from build123d import *

# Parameters (mm, degrees)
CHAMFER_1_SIZE = 1
CHAMFER_2_SIZE = 1
FILLET_1_R     = 0.2


with BuildPart() as part:
    # 스케치3 → 회전2 (revolve)
    with BuildSketch(Plane(origin=(0, 0, 0), x_dir=(1, 0, 0), z_dir=(0, 1, 0)), mode=Mode.PRIVATE) as revolve_2_sk:
        Polygon((11.1, 0), (11.1, -2.4), (8.6, -2.4), (8.6, -4.2), (11.1, -6.2), (11.1, -8.2), (10, -8.2), (10, -10.2), (9.5, -10.7), (9.5, -11.2), (10, -11.7), (10, -12.2), (9.5, -12.7), (9.5, -13.2), (10, -13.7), (10, -14.2), (9.5, -14.7), (9.5, -15.2), (10, -15.7), (10, -16.2), (9.5, -16.7), (9.5, -17.2), (10, -17.7), (10, -19.8), (2.9, -19.8), (2.9, -11.8), (4.4, -11.8), (4.4, -10), (3.4, -10), (3.4, -8.5), (6.25, -7.736344802), (6.25, 0), align=None)
    revolve(revolve_2_sk.sketch.rotate(Axis((0, 0, 0), (0, 0, 1)), 180), axis=Axis((0, 0, 0), (0, 0, 1)))

    # 모따기1
    chamfer_1_edges = [part.edges().sort_by_distance(p)[0] for p in [
        (10, 0, 19.8),
        (6.25, 0, 0),
    ]]
    chamfer(chamfer_1_edges, length=CHAMFER_1_SIZE)

    # 모따기2
    chamfer_2_edges = [part.edges().sort_by_distance(p)[0] for p in [
        (11.1, 0, 0),
    ]]
    chamfer(chamfer_2_edges, length=CHAMFER_2_SIZE)

    # 필렛1
    fillet_1_edges = [part.edges().sort_by_distance(p)[0] for p in [
        (11.1, 0, 2.4),
    ]]
    fillet(fillet_1_edges, radius=FILLET_1_R)


solid = part.part
Could you check a few things on this model? Use its own coordinates, in mm. A direction names the side the tool comes from. Give positions to 0.01 mm unless a question says otherwise; leave off trailing zeros. Write each loop counter-clockwise with the first axis right and the second up, starting at its lowest first coordinate (ties: lowest second). Pieces come first, ordered by that corner, then holes. Notation, with made-up numbers: (-25, 23.25) -> (-6, 23.25) arc R26 cw to (-6, 45.25) -> close; hole circle Ø1 at (-33.75, -15.5). An arc over 180 degrees is marked (long way). Answer as CSV lines item,"result". Start each with the question number.
(1) I'm going to push flat-ended pins straight in: pin 1 Ø5 at (y, z) = (8, 11.5) entering from -X; pin 2 Ø5 at (y, z) = (-7, 14.5) entering from -X; pin 3 Ø4.5 at (x, y) = (2, 1.5) entering from -Z. Where does each tip first touch, or does it pass through?
(2) Which directions (+Z, -Z, +X, -X, +Y, -Y) give clear straight access to the entire face, cutting with the end or side of a thin tool? Please do faces 4 (the face through (1.445, -11.006, 7.214)), 5 (the face through (10, 0, 14)), 6 (the face through (-5.96, -1.88, 4.32)), 7 (the face through (2.059, 9.274, 16.954)).
(3) If we section it at A-A, the plane z = 5: Write out the boundary of the cut face in (x, y), and give its area (3 significant figures).
(4) If we mould it in two halves opening along X, with no side actions, what happens to faces 1 (the face through (0.74, 3.32, 9.24)), 2 (the face through (10, 0, 18)), 3 (the face through (0, 4, 19.8))? For each: +X half, -X half, draft (parallel to the pull), parting line (faces both ways), or undercut.
(5) Please list where these lines run through material, in increasing order: line 1 (Y direction, x = 0, z = 9.5); line 2 (Y direction, x = 0, z = 11.2); line 3 (X direction, y = 3, z = 11.25).
Answer list:
1,pin 1,"x = -8.35"
1,pin 2,"x = -8.92"
1,pin 3,"z = 8.14"
2,face 4,"+Z, -Z"
2,face 5,"+Z"
2,face 6,"-Z"
2,face 7,"none"
3,outline,"circle Ø19.2 at (0, 0); hole circle Ø12.5 at (0, 0)"
3,area,"167 mm^2"
4,face 1,"undercut"
4,face 2,"parting line"
4,face 3,"draft"
5,line 1,"-10 to -3.4, 3.4 to 10"
5,line 2,"-9.5 to -4.4, 4.4 to 9.5"
5,line 3,"-9.07 to -3.22, 3.22 to 9.07"
